Could you check a few things on this model? Use its own coordinates, in mm. A direction names the side the tool comes from. Give positions to 0.01 mm unless a question says otherwise; leave off trailing zeros. Write each loop counter-clockwise with the first axis right and the second up, starting at its lowest first coordinate (ties: lowest second). Pieces come first, ordered by that corner, then holes. Notation, with made-up numbers: M -4.5,-24 L 44.5,-24 A15 ccw 44.5,1 Z; hole C 88,78 d6. An arc over 180 degrees is marked long. Answer as CSV lines item,"result". Start each with the question number.
from build123d import *

# Parameters (mm, degrees)
SKETCH_1_W           = 50
SKETCH_1_H           = 39.5
SKETCH_1_R           = 1.51
SKETCH_1_R_2         = 1.75
SKETCH_1_R_3         = 3
EXTRUDE_1_DEPTH      = 2.5
SKETCH_2_W           = 2
SKETCH_2_H           = 39.5
EXTRUDE_6_DEPTH      = 28
SKETCH_3_W           = 50
SKETCH_3_H           = 39.5
SKETCH_3_R           = 1.75
SKETCH_3_R_2         = 3
SKETCH_3_R_3         = 1.51
EXTRUDE_7_DEPTH      = 2.5
SKETCH_4_W           = 16.941744986
SKETCH_4_H           = 9.266793399
CUT_EXTRUDE_1_DEPTH  = 10
SKETCH_5_W           = 6.8
SKETCH_5_H           = 39.5
EXTRUDE_8_DEPTH      = 29
SKETCH_6_OUTSIDE_W   = 70.584
SKETCH_6_OUTSIDE_H   = 45.584
SKETCH_6_OUTSIDE_W_2 = 45.4
SKETCH_6_OUTSIDE_H_2 = 28
CUT_EXTRUDE_2_DEPTH  = 55.217155956
SKETCH_7_R           = 1.25
CUT_EXTRUDE_3_DEPTH  = 10
SKETCH_8_R           = 2
CUT_EXTRUDE_4_DEPTH  = 1.5
SKETCH_9_W           = 16.827913255
SKETCH_9_H           = 6.559808616
CUT_EXTRUDE_5_DEPTH  = 10


with BuildPart() as part:
    # 草图1 → 凸台-拉伸1 (new body)
    with BuildSketch(Plane(origin=(0, 0, 0), x_dir=(1, 0, 0), z_dir=(0, 1, 0))):
        Rectangle(SKETCH_1_W, SKETCH_1_H)
        with Locations(Location((22.5, 9.75, 0), (0, 0, 270))):
            Circle(SKETCH_1_R, mode=Mode.SUBTRACT)
        with Locations(Location((-22.5, 9.75, 0), (0, 0, 270))):
            Circle(SKETCH_1_R, mode=Mode.SUBTRACT)
        with Locations(Location((-5, -5, 0), (0, 0, 270))):
            Circle(SKETCH_1_R_2, mode=Mode.SUBTRACT)
        with Locations(Location((5, -5, 0), (0, 0, 270))):
            Circle(SKETCH_1_R_2, mode=Mode.SUBTRACT)
        with Locations(Location((5, 5, 0), (0, 0, 270))):
            Circle(SKETCH_1_R_2, mode=Mode.SUBTRACT)
        with Locations(Location((-5, 5, 0), (0, 0, 270))):
            Circle(SKETCH_1_R_2, mode=Mode.SUBTRACT)
        with Locations(Location((0, 0, 0), (0, 0, 270))):
            Circle(SKETCH_1_R_3, mode=Mode.SUBTRACT)
        with Locations(Location((22.5, -9.75, 0), (0, 0, 270))):
            Circle(SKETCH_1_R, mode=Mode.SUBTRACT)
        with Locations(Location((-22.5, -9.75, 0), (0, 0, 270))):
            Circle(SKETCH_1_R, mode=Mode.SUBTRACT)
    extrude(amount=EXTRUDE_1_DEPTH)

    # 草图2 → 凸台-拉伸6 (add)
    with BuildSketch(Plane(origin=(0, 2.5, 0), x_dir=(1, 0, 0), z_dir=(0, 1, 0))):
        with Locations((-26, 0)):
            Rectangle(SKETCH_2_W, SKETCH_2_H)
        with Locations((26, 0)):
            Rectangle(SKETCH_2_W, SKETCH_2_H)
    extrude(amount=-EXTRUDE_6_DEPTH)

    # 草图3 → 凸台-拉伸7 (add)
    with BuildSketch(Plane.XZ.offset(25.5)):
        Rectangle(SKETCH_3_W, SKETCH_3_H)
        with Locations(Location((-5, 5, 0), (0, 0, 90))):
            Circle(SKETCH_3_R, mode=Mode.SUBTRACT)
        with Locations(Location((5, 5, 0), (0, 0, 90))):
            Circle(SKETCH_3_R, mode=Mode.SUBTRACT)
        with Locations(Location((5, -5, 0), (0, 0, 90))):
            Circle(SKETCH_3_R, mode=Mode.SUBTRACT)
        with Locations(Location((-5, -5, 0), (0, 0, 90))):
            Circle(SKETCH_3_R, mode=Mode.SUBTRACT)
        with Locations(Location((0, 0, 0), (0, 0, 90))):
            Circle(SKETCH_3_R_2, mode=Mode.SUBTRACT)
        with Locations(Location((22.5, -9.75, 0), (0, 0, 90))):
            Circle(SKETCH_3_R_3, mode=Mode.SUBTRACT)
        with Locations(Location((-22.5, -9.75, 0), (0, 0, 90))):
            Circle(SKETCH_3_R_3, mode=Mode.SUBTRACT)
        with Locations(Location((-22.5, 9.75, 0), (0, 0, 90))):
            Circle(SKETCH_3_R_3, mode=Mode.SUBTRACT)
        with Locations(Location((22.5, 9.75, 0), (0, 0, 90))):
            Circle(SKETCH_3_R_3, mode=Mode.SUBTRACT)
    extrude(amount=-EXTRUDE_7_DEPTH)

    # 草图4 → 切除-拉伸1 (cut)
    with BuildSketch(Plane.XZ.offset(25.5)):
        with Locations((-10.403823263, -13.116741256)):
            Rectangle(SKETCH_4_W, SKETCH_4_H)
    extrude(amount=-CUT_EXTRUDE_1_DEPTH, mode=Mode.SUBTRACT)

    # 草图5 → 凸台-拉伸8 (add)
    with BuildSketch(Plane.XZ.offset(25.5)):
        with Locations((23.6, 0)):
            Rectangle(SKETCH_5_W, SKETCH_5_H)
        with Locations((-23.6, 0)):
            Rectangle(SKETCH_5_W, SKETCH_5_H)
    extrude(amount=-EXTRUDE_8_DEPTH)

    # 草图6 outside → 切除-拉伸2 (cut, through all)
    with BuildSketch(Plane.XY.offset(19.75)):
        with Locations((0, -11)):
            Rectangle(SKETCH_6_OUTSIDE_W, SKETCH_6_OUTSIDE_H)
        with Locations((0, -11.5)):
            Rectangle(SKETCH_6_OUTSIDE_W_2, SKETCH_6_OUTSIDE_H_2, mode=Mode.SUBTRACT)
    extrude(amount=-CUT_EXTRUDE_2_DEPTH, mode=Mode.SUBTRACT)

    # 草图7 → 切除-拉伸3 (cut)
    with BuildSketch(Plane(origin=(0, 2.5, 0), x_dir=(1, 0, 0), z_dir=(0, 1, 0))):
        with Locations(Location((14.15, 14.15, 0), (0, 0, 270))):
            Circle(SKETCH_7_R)
        with Locations(Location((14.15, -14.15, 0), (0, 0, 270))):
            Circle(SKETCH_7_R)
        with Locations(Location((-14.15, -14.15, 0), (0, 0, 270))):
            Circle(SKETCH_7_R)
        with Locations(Location((-14.15, 14.15, 0), (0, 0, 270))):
            Circle(SKETCH_7_R)
    extrude(amount=-CUT_EXTRUDE_3_DEPTH, mode=Mode.SUBTRACT)

    # 草图8 → 切除-拉伸4 (cut)
    with BuildSketch(Plane.XZ):
        with Locations(Location((-14.15, -14.15, 0), (0, 0, 270))):
            Circle(SKETCH_8_R)
        with Locations(Location((-14.15, 14.15, 0), (0, 0, 270))):
            Circle(SKETCH_8_R)
        with Locations(Location((14.15, 14.15, 0), (0, 0, 270))):
            Circle(SKETCH_8_R)
        with Locations(Location((14.15, -14.15, 0), (0, 0, 270))):
            Circle(SKETCH_8_R)
    extrude(amount=-CUT_EXTRUDE_4_DEPTH, mode=Mode.SUBTRACT)

    # 草图9 → 切除-拉伸5 (cut)
    with BuildSketch(Plane(origin=(0, 2.5, 0), x_dir=(1, 0, 0), z_dir=(0, 1, 0))):
        with Locations((-14.286043373, -13.437027327)):
            Rectangle(SKETCH_9_W, SKETCH_9_H)
    extrude(amount=-CUT_EXTRUDE_5_DEPTH, mode=Mode.SUBTRACT)


solid = part.part
1. Please list where these lines run through material, in increasing order: line 1 (X direction, y = -24.8, z = -5); line 2 (Y direction, x = 11, z = -7); line 3 (X direction, y = -21.5, z = -10.5).
2. Will these pins go through, and if not, where does the flat tip stop? P1, Ø4, axis at x = 5, z = 5, coming from the +Y side; P2, Ø5, axis at x = 0, z = 0, coming from the +Y side; P3, Ø0.8, axis at x = -21.5, z = 12.5, coming from the +Y side.
3. Imagine slicing it at D-D, the plane z = 14.15. Please give me the cut outline in (x, y), plus the area to 3 significant figures.
4. Imagine slicing it at A-A, the plane z = -14.15. Please give me the cut outline in (x, y).
5. On a 3-axis mill with a long thin cutter (end or side, diameter ignored), from which of +Z, -Z, +X, -X, +Y, -Y can I reach the whole of each face in a straight line? I mean faces 1 (the flat face through (13, 1.5, -13)), 2 (the flat face through (-21, -7.5, 13)), 3 (the cylindrical face through (-13.549, 0.74, -16.058)), 4 (the flat face through (0, 0, -5)), 5 (the cylindrical face through (13.041, 2.007, 14.727)). Say none if no direction works.
6. Imagine slicing it at B-B, the plane x = -19.5. Please give me the cut outline in (y, z).
7. Thinking about a two-plate mould opening in X: for faces 6 (the flat face through (-5, 1, -19.75)), 7 (the cylindrical face through (14.751, 0.74, -16.058)), which applies, pulls with the +X half, pulls with the -X half, needs draft (parallel to the pull), parting line crosses it, or undercut?
8. Imagine slicing it at C-C, the plane y = -24. Please give me the cut outline in (x, z), plus the area to 3 significant figures.
Solutions:
1,line 1,"-22.7 to -6.75, -3.25 to 3.25, 6.75 to 22.7"
1,line 2,"-25.5 to -23, 0 to 2.5"
1,line 3,"-22.7 to -20.2, 20.2 to 22.7"
2,P1,"y = 2.5"
2,P2,"through"
2,P3,"y = -7.5"
3,outline,"M -22.7,-25.5 L 22.7,-25.5 L 22.7,2.5 L 15.4,2.5 L 15.4,1.5 L 16.15,1.5 L 16.15,0 L 20.2,0 L 20.2,-23 L -20.2,-23 L -20.2,-7.5 L -22.7,-7.5 Z; M -5.87,0 L 12.15,0 L 12.15,1.5 L 12.9,1.5 L 12.9,2.5 L -5.87,2.5 Z"
3,area,"273 mm²"
4,outline,"M -22.7,-25.5 L -18.87,-25.5 L -18.87,-23 L -20.2,-23 L -20.2,0 L -16.15,0 L -16.15,1.5 L -15.4,1.5 L -15.4,2.5 L -22.7,2.5 Z; M -12.9,1.5 L -12.15,1.5 L -12.15,0 L 12.15,0 L 12.15,1.5 L 12.9,1.5 L 12.9,2.5 L -12.9,2.5 Z; M -1.93,-25.5 L 22.7,-25.5 L 22.7,2.5 L 15.4,2.5 L 15.4,1.5 L 16.15,1.5 L 16.15,0 L 20.2,0 L 20.2,-23 L -1.93,-23 Z"
5,face 1,"none"
5,face 2,"-X, +Y"
5,face 3,"-Y"
5,face 4,"+Z, -Z"
5,face 5,"+Y"
6,outline,"M -25.5,-19.75 L -23,-19.75 L -23,19.75 L -25.5,19.75 Z; M 0,-19.75 L 2.5,-19.75 L 2.5,10.16 L 0,10.16 Z; M 0,16.72 L 2.5,16.72 L 2.5,19.75 L 0,19.75 Z"
7,face 6,"needs draft"
7,face 7,"undercut"
8,outline,"M -22.7,-19.75 L 22.7,-19.75 L 22.7,19.75 L -22.7,19.75 Z; hole M -18.87,-17.75 L -1.93,-17.75 L -1.93,-8.48 L -18.87,-8.48 Z; hole C -5,-5 d3.5; hole C -5,5 d3.5; hole C 0,0 d6; hole C 5,-5 d3.5; hole C 5,5 d3.5"
8,area,"1,570 mm²"
